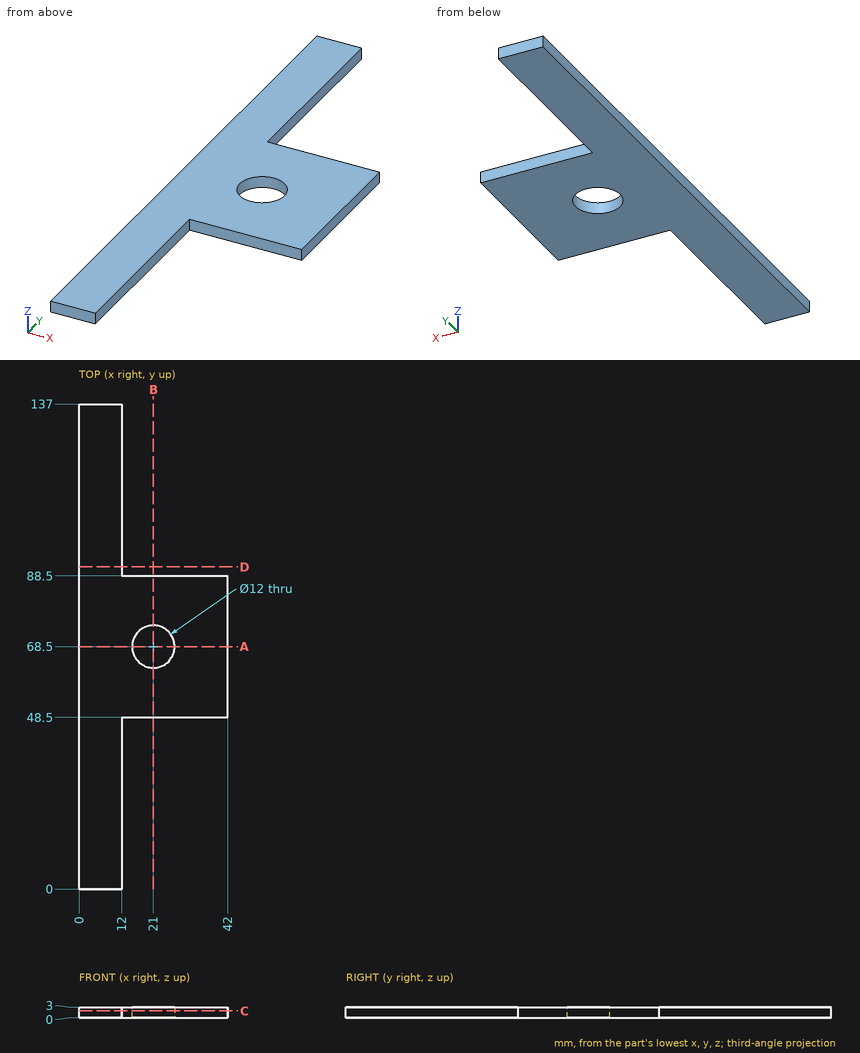
Job drawing, mm, ordinate dimensions from the low corner. One solid piece. Coordinates: 2 decimals unless noted, no trailing zeros. Write each loop counter-clockwise with the first axis right and the second up, starting at its lowest first coordinate (ties: lowest second). Pieces come first, ordered by that corner, then holes.
Item 1: Pin check, flat tip, straight feed: pin 1 (1 mm diameter, centred on x = 35.5, z = 0.5, fed in from +Y). Stop position of the tip, or through.
Item 2: Slice it at A-A (y = 68.5). Write the cut outline in (x, z), and give its area (3 significant figures).
Item 3: Slice it at C-C (z = 2). Write the cut outline in (x, y).
Item 4: Slice it at B-B (x = 21). Write the cut outline in (y, z), and give its area (3 significant figures).
Item 5: Probe line 1 (Y direction, x = 21, z = 1.35); line 2 (X direction, y = 109, z = 0.4); line 3 (Y direction, x = 19, z = 1.25). List the from-to ranges inside material, lowest first.
Item 6: Slice it at D-D (y = 91). Write the cut outline in (x, z), and give its area (3 significant figures).
Results found:
1. pin 1: stops at y = 88.5
2. outline: (0, 0) - (15, 0) - (15, 3) - (0, 3) - close; (27, 0) - (42, 0) - (42, 3) - (27, 3) - close
2. area: 90.0 mm2
3. outline: (0, 0) - (12, 0) - (12, 48.5) - (42, 48.5) - (42, 88.5) - (12, 88.5) - (12, 137) - (0, 137) - close; hole circle Ø12 at (21, 68.5)
4. outline: (48.5, 0) - (62.5, 0) - (62.5, 3) - (48.5, 3) - close; (74.5, 0) - (88.5, 0) - (88.5, 3) - (74.5, 3) - close
4. area: 84.0 mm2
5. line 1: y = 48.5 to 62.5, 74.5 to 88.5
5. line 2: x = 0 to 12
5. line 3: y = 48.5 to 62.84, 74.16 to 88.5
6. outline: (0, 0) - (12, 0) - (12, 3) - (0, 3) - close
6. area: 36.0 mm2
